from build123d import *

# Parameters (mm, degrees)
SKETCH_1_R          = 2
EXTRUDE_1_DEPTH     = 8
SKETCH_2_R          = 3.5
EXTRUDE_2_DEPTH     = 4
CUT_EXTRUDE_1_DEPTH = 2
FILLET_1_R          = 0.2


with BuildPart() as part:
    # 草图1 → 凸台-拉伸1 (new body)
    with BuildSketch(Plane.XY):
        Circle(SKETCH_1_R)
    extrude(amount=EXTRUDE_1_DEPTH)

    # 草图2 → 凸台-拉伸2 (add)
    with BuildSketch(Plane.XY):
        Circle(SKETCH_2_R)
    extrude(amount=-EXTRUDE_2_DEPTH)

    # 草图3 → 切除-拉伸1 (cut)
    with BuildSketch(Plane(origin=(0, 0, -4), x_dir=(-1, 0, 0), z_dir=(0, 0, -1))):
        Polygon((0, 1.72), (-1.5, 0.863623327), (-1.5, -0.863623327), (0, -1.72), (1.5, -0.863623327), (1.5, 0.863623327), align=None)
    extrude(amount=-CUT_EXTRUDE_1_DEPTH, mode=Mode.SUBTRACT)

    # 圆角1
    fillet_1_edges = [part.edges().sort_by_distance(p)[0] for p in [
        (-3.5, 0, -4),
    ]]
    fillet(fillet_1_edges, radius=FILLET_1_R)


solid = part.part
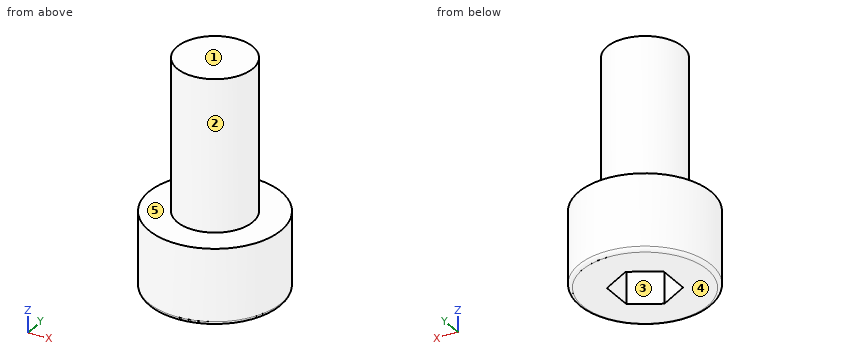
Read the model definition and answer for the solid it produces. Units are mm, in the model's axes. Face numbers are marked on the shaded views. A direction names the side the tool comes from. Round coordinates to 2 decimals unless told otherwise and drop trailing zeros. Write each loop counter-clockwise with the first axis right and the second up, starting at its lowest first coordinate (ties: lowest second). Pieces come first, ordered by that corner, then holes. Notation, with made-up numbers: M -31,83.5 L -22,83.5 A18 ccw -22,101.5 Z; hole C 5,15 d6. An arc over 180 degrees is marked long. Use a Markdown table: item, result.
1) The part is cut by section B-B (z = -2.5). Write down the section's boundary in (x, y), plus the area to 3 significant figures.
Answers follow:
| item | result |
|---|---|
| outline | C 0,0 d7; hole M -1.5,-0.86 L 0,-1.72 L 1.5,-0.86 L 1.5,0.86 L 0,1.72 L -1.5,0.86 Z |
| area | 30.7 mm2 |
2) A tool of negligible diameter and unlimited length cuts with its end or side. For the marked faces 4 and 5, from which of +Z, -Z, +X, -X, +Y, -Y can it reach the whole face along a straight path? Write none if from no direction.
Answers follow:
| item | result |
|---|---|
| face 4 | -Z, +X, -X, +Y, -Y |
| face 5 | +Z |
3) The part is cut by section C-C (z = 3.25). Write down the section's boundary in (x, y).
Answers follow:
| item | result |
|---|---|
| outline | C 0,0 d4 |
4) Flat-ended cylindrical pins translate along their axes: pin 1 (2 mm diameter, centred on y = -2, z = 5, fed in from +X); pin 2 (4 mm diameter, centred on x = 1.5, z = 3.5, fed in from +Y); pin 3 (1 mm diameter, centred on y = -2, z = 3.5, fed in from +X). Find the tip coordinate at first contact, or state that the pin passes through.
Answers follow:
| item | result |
|---|---|
| pin 1 | stops at x = 1.73 |
| pin 2 | stops at y = 2 |
| pin 3 | stops at x = 1.32 |
5) The part is cut by section A-A (y = 0). Write down the section's boundary in (x, z).
Answers follow:
| item | result |
|---|---|
| outline | M -3.5,-3.8 A0.2 ccw -3.3,-4 L -1.5,-4 L -1.5,-2 L 1.5,-2 L 1.5,-4 L 3.3,-4 A0.2 ccw 3.5,-3.8 L 3.5,0 L 2,0 L 2,8 L -2,8 L -2,0 L -3.5,0 Z |
6) Straight lines are drawn through the part: line 1 along Z through (x, y) = (0, -1); line 2 along X through (y, z) = (1.5, -3); line 3 along Z through (x, y) = (1.75, 2). For each, find the intervals that lie inside material, in ascending order. Write a range as [from, to].
Answers follow:
| item | result |
|---|---|
| line 1 | z = [-2, 8] |
| line 2 | x = [-3.16, -0.39], [0.39, 3.16] |
| line 3 | z = [-4, 0] |
7) For a pull along Y with two mould halves and no side action, classify the marked faces 1, 2 and 3 as pulls with the +Y half, pulls with the -Y half, needs draft (parallel to the pull), parting line crosses it, or undercut.
Answers follow:
| item | result |
|---|---|
| face 1 | needs draft |
| face 2 | parting line crosses it |
| face 3 | undercut |
